CAD build for the part. Positions are in the model's coordinates, mm. Face numbers are marked on the shaded views. A direction names the side the tool comes from. Give positions to 0.01 mm unless a question says otherwise; leave off trailing zeros. Order: outer loops, then holes, each group sorted by start corner. A loop starts at its lowest first (then second) coordinate and runs counter-clockwise, first axis right, second up. Notation, with made-up numbers: M 53,63.5 L 91,63.5 A28 ccw 91,90.5 Z; hole C 59,36.25 d3. An arc over 180 degrees is marked long. Put each result on its own line as item: value. Start each with the question number.
1) Cut at D-D (y = 17). Write the cut outline in (x, z), and give its area (3 significant figures).
2) Cut at C-C (y = -16.4). Write the cut outline in (x, z).
3) Drill centre lines: line 1 (Y direction, x = -6.05, z = 1); line 2 (Y direction, x = -7, z = 5.25); line 3 (X direction, y = -1.5, z = 14). Where is each one in solid material? Low to high. Write a range as [from, to].
4) Two-plate mould, pull along X, no slides. Class the marked faces 4, 5, 6 and 7: released by +X, released by -X, zero draft, split by the parting line, or undercut.
5) Pin check, flat tips, straight feed: pin 1 (3 mm diameter, centred on x = -6.05, y = -16.4, fed in from +Z); pin 2 (6.5 mm diameter, centred on x = -5, y = -5, fed in from +Z); pin 3 (1 mm diameter, centred on x = 0, y = -13, fed in from -Z); pin 4 (0.8 mm diameter, centred on x = 2, z = 1, fed in from +Y). Stop position of each tip, or through.
6) Cut at B-B (z = 15). Write the cut outline in (x, y), and give its area (3 significant figures).
7) Tool access for the marked faces 1, 2 and 3: list every direction of +Z, -Z, +X, -X, +Y, -Y with a clear straight run to the whole face (end or side of a thin tool).
8) Cut at A-A (x = 6.05). Write the cut outline in (y, z).
```python
from build123d import *

# Parameters (mm, degrees)
CROQUIS1_W              = 20
CROQUIS1_H              = 37.5
CROQUIS1_R              = 1.35
SALIENTE_EXTRUIR1_DEPTH = 1.5
CROQUIS2_W              = 16.8
CROQUIS2_H              = 11.6
SALIENTE_EXTRUIR2_DEPTH = 2.3
CROQUIS3_W              = 16.8
CROQUIS3_H              = 13.9
SALIENTE_EXTRUIR3_DEPTH = 12.4
CROQUIS4_W              = 6.1
CROQUIS4_H              = 15.2
SALIENTE_EXTRUIR4_DEPTH = 14.6


with BuildPart() as part:
    # Croquis1 → Saliente-Extruir1 (new body)
    with BuildSketch(Plane.XY):
        Rectangle(CROQUIS1_W, CROQUIS1_H)
        with Locations((-6.05, -16.4)):
            Circle(CROQUIS1_R, mode=Mode.SUBTRACT)
        with Locations((6.05, -16.4)):
            Circle(CROQUIS1_R, mode=Mode.SUBTRACT)
    extrude(amount=SALIENTE_EXTRUIR1_DEPTH)

    # Croquis2 → Saliente-Extruir2 (add)
    with BuildSketch(Plane.XY.offset(1.5)):
        with Locations((0, 14.25)):
            Rectangle(CROQUIS2_W, CROQUIS2_H)
    extrude(amount=SALIENTE_EXTRUIR2_DEPTH)

    # Croquis3 → Saliente-Extruir3 (add)
    with BuildSketch(Plane.XY.offset(3.8)):
        with Locations((0, 15.4)):
            Rectangle(CROQUIS3_W, CROQUIS3_H)
    extrude(amount=SALIENTE_EXTRUIR3_DEPTH)

    # Croquis4 → Saliente-Extruir4 (add)
    with BuildSketch(Plane.XY.offset(1.5)):
        with Locations((-6.65, -6.95)):
            Rectangle(CROQUIS4_W, CROQUIS4_H)
        with Locations((6.65, -6.95)):
            Rectangle(CROQUIS4_W, CROQUIS4_H)
    extrude(amount=SALIENTE_EXTRUIR4_DEPTH)


solid = part.part
```
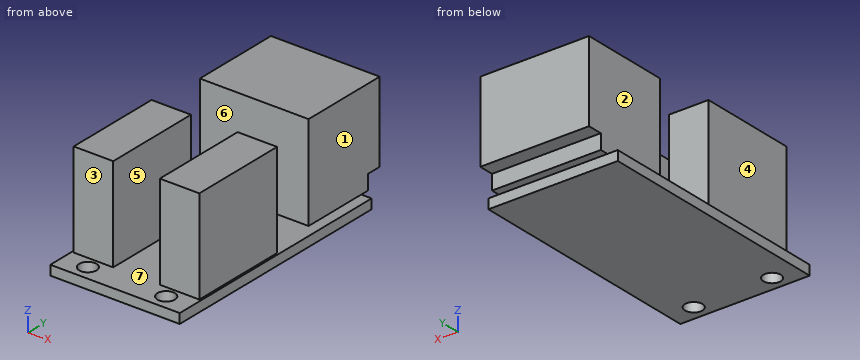
Solution:
1. outline: M -10,0 L 10,0 L 10,1.5 L 8.4,1.5 L 8.4,16.2 L -8.4,16.2 L -8.4,1.5 L -10,1.5 Z
1. area: 277 mm²
2. outline: M -10,0 L -7.4,0 L -7.4,1.5 L -10,1.5 Z; M -4.7,0 L 4.7,0 L 4.7,1.5 L -4.7,1.5 Z; M 7.4,0 L 10,0 L 10,1.5 L 7.4,1.5 Z
3. line 1: [-18.75, -17.75], [-15.05, 18.75]
3. line 2: [-14.55, 0.65], [8.45, 22.35]
3. line 3: [-9.7, -3.6], [3.6, 9.7]
4. face 4: released by -X
4. face 5: undercut
4. face 6: zero draft
4. face 7: undercut
5. pin 1: z = 1.5
5. pin 2: z = 16.1
5. pin 3: z = 0
5. pin 4: y = 18.75
6. outline: M -9.7,-14.55 L -3.6,-14.55 L -3.6,0.65 L -9.7,0.65 Z; M -8.4,8.45 L 8.4,8.45 L 8.4,22.35 L -8.4,22.35 Z; M 3.6,-14.55 L 9.7,-14.55 L 9.7,0.65 L 3.6,0.65 Z
6. area: 419 mm²
7. face 1: +Z, +X, +Y
7. face 2: +Z, -X, +Y
7. face 3: +Z, +X, -X, -Y
8. outline: M -18.75,0 L -17.75,0 L -17.75,1.5 L -18.75,1.5 Z; M -15.05,0 L 18.75,0 L 18.75,1.5 L 20.05,1.5 L 20.05,3.8 L 22.35,3.8 L 22.35,16.2 L 8.45,16.2 L 8.45,1.5 L 0.65,1.5 L 0.65,16.1 L -14.55,16.1 L -14.55,1.5 L -15.05,1.5 Z
